Could you check a few things on this model? Use its own coordinates, in mm. Face numbers are marked on the shaded views. A direction names the side the tool comes from. Give positions to 0.01 mm unless a question says otherwise; leave off trailing zeros. Write each loop counter-clockwise with the first axis right and the second up, starting at its lowest first coordinate (ties: lowest second). Pieces come first, ordered by that corner, then holes. Notation, with made-up numbers: M 43,78 L 68,78 A26 cw 68,116 Z; hole C 37.25,5 d9. An arc over 180 degrees is marked long. Answer as CSV lines item,"result". Start each with the question number.
from build123d import *

# Parameters (mm, degrees)
BASE_W              = 500
BASE_H              = 300
EXTRUDE_1_DEPTH     = 120
SKETCH_1_W          = 480
SKETCH_1_H          = 110
CUT_EXTRUDE_1_DEPTH = 596.315042645
CUT_EXTRUDE_2_DEPTH = 596.315042645
SKETCH_3_W          = 200
SKETCH_3_H          = 105
SKETCH_3_W_2        = 10
CUT_EXTRUDE_3_DEPTH = 596.315042645


with BuildPart() as part:
    # base → 凸台-拉伸1 (new body)
    with BuildSketch(Plane(origin=(0, 0, 0), x_dir=(1, 0, 0), z_dir=(0, 1, 0))):
        with Locations((250, -150)):
            Rectangle(BASE_W, BASE_H)
    extrude(amount=EXTRUDE_1_DEPTH)

    # 草图1 → 切除-拉伸1 (cut, through all)
    with BuildSketch(Plane(origin=(0, 0, 0), x_dir=(-1, 0, 0), z_dir=(0, 0, -1))):
        with Locations((-250, 65)):
            Rectangle(SKETCH_1_W, SKETCH_1_H)
    extrude(amount=-CUT_EXTRUDE_1_DEPTH, mode=Mode.SUBTRACT)

    # 草图2 → 切除-拉伸2 (cut, through all)
    with BuildSketch(Plane.XZ):
        Polygon((10, 280), (10, 20), (236.296296296, 150), align=None)
        Polygon((20, 290), (480, 290), (250, 157.872340426), align=None)
        Polygon((263.703703704, 150), (490, 280), (490, 20), align=None)
        Polygon((250, 142.127659574), (20, 10), (480, 10), align=None)
    extrude(amount=-CUT_EXTRUDE_2_DEPTH, mode=Mode.SUBTRACT)

    # 草图3 → 切除-拉伸3 (cut, through all)
    with BuildSketch(Plane.ZY):
        with Locations((150, 67.5)):
            Rectangle(SKETCH_3_W, SKETCH_3_H)
        with Locations((5, 67.5)):
            Rectangle(SKETCH_3_W_2, SKETCH_3_H)
        with Locations((295, 67.5)):
            Rectangle(SKETCH_3_W_2, SKETCH_3_H)
    extrude(amount=-CUT_EXTRUDE_3_DEPTH, mode=Mode.SUBTRACT)


solid = part.part
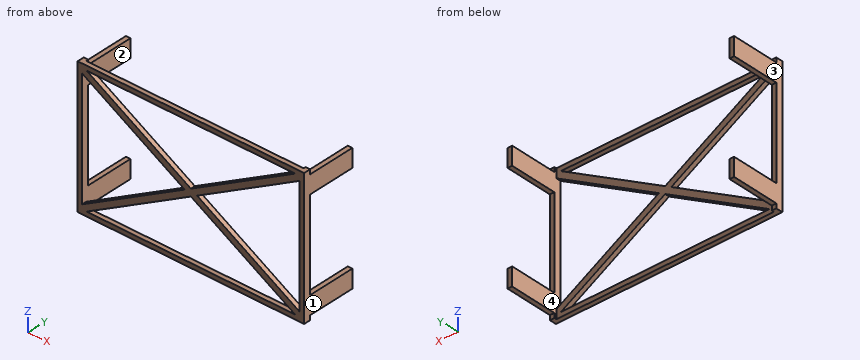
1. On a 3-axis mill with a long thin cutter (end or side, diameter ignored), from which of +Z, -Z, +X, -X, +Y, -Y can I reach the whole of each face in a straight line? I mean the marked faces 3 and 4. Say none if no direction works.
2. Thinking about a two-plate mould opening in Z: for the marked faces 1 and 2, which applies, pulls with the +Z half, pulls with the -Z half, needs draft (parallel to the pull), parting line crosses it, or undercut?
3. Imagine slicing it at C-C, the plane x = 242.5. Please give me the cut outline in (y, z).
4. Will these pins go through, and if not, where does the flat tip stop? P1, Ø5, axis at x = 497, y = 74, coming from the +Z side; P2, Ø5, axis at x = 3, y = 57, coming from the -Z side; P3, Ø8, axis at x = 6.5, z = 297, coming from the +Y side; P4, Ø3, axis at x = 310.5, y = 6, coming from the -Z side.
5. Imagine slicing it at A-A, the plane y = 22. Please give me the cut outline in (x, z), plus the area to 3 significant figures.
6. Please list where these lines run through material, in increasing order: line 1 (X direction, y = 43.5, z = 36.5); line 2 (X direction, y = 6, z = 259); line 3 (Y direction, x = 394.5, z = 226).
7. Imagine slicing it at B-B, the plane x = 118.5. Please give me the cut outline in (y, z), plus the area to 3 significant figures.
Solutions:
1,face 3,"+Z, -Z, -X, +Y, -Y"
1,face 4,"+Y"
2,face 1,"needs draft"
2,face 2,"undercut"
3,outline,"M 0,0 L 10,0 L 10,10 L 0,10 Z; M 0,137.82 L 10,137.82 L 10,162.18 L 0,162.18 Z; M 0,290 L 10,290 L 10,300 L 0,300 Z"
4,P1,"z = 290"
4,P2,"z = 10"
4,P3,"y = 15"
4,P4,"z = 0"
5,outline,"M 0,10 L 10,10 L 10,50 L 0,50 Z; M 0,250 L 10,250 L 10,290 L 0,290 Z; M 490,10 L 500,10 L 500,50 L 490,50 Z; M 490,250 L 500,250 L 500,290 L 490,290 Z"
5,area,"1,600 mm²"
6,line 1,"0 to 10, 490 to 500"
6,line 2,"0 to 10, 46.56 to 73.96, 426.04 to 453.44, 490 to 500"
6,line 3,"0 to 10"
7,outline,"M 0,0 L 10,0 L 10,10 L 0,10 Z; M 0,66.59 L 10,66.59 L 10,82.33 L 0,82.33 Z; M 0,217.67 L 10,217.67 L 10,233.41 L 0,233.41 Z; M 0,290 L 10,290 L 10,300 L 0,300 Z"
7,area,"515 mm²"
